For this review, use the dimensioned drawing (mm, ordinates from the lowest corner) and the shaded views. Coordinates: 2 decimals unless noted, no trailing zeros. Write each loop counter-clockwise with the first axis right and the second up, starting at its lowest first coordinate (ties: lowest second). Pieces come first, ordered by that corner, then holes. Notation, with made-up numbers: (2, 80.5) - (33, 80.5) arc R22 ccw to (33, 87.5) - close; hole circle Ø5 at (29.25, 29). An arc over 180 degrees is marked (long way). One line per item, written item: value.
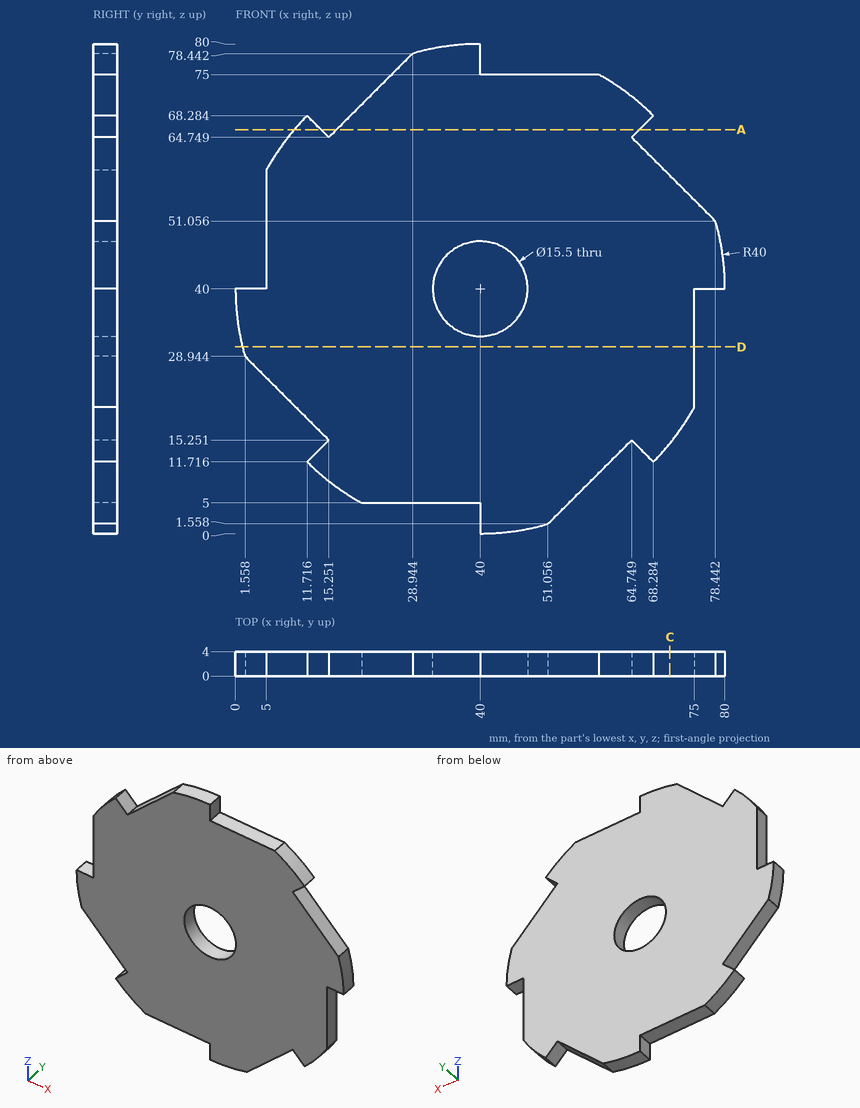
1. Consider section D-D, the plane z = 30.5. Write out the cut boundary in (x, y) (1 decimal).
Answer block:
outline: (1.1, 0) - (75, 0) - (75, 4) - (1.1, 4) - close
2. Insertion check: pin 1 Ø2 at (y, z) = (1.5, 52) entering from -X; pin 2 Ø1 at (x, y) = (36.5, 2.5) entering from -Z; pin 3 Ø1.2 at (y, z) = (1.5, 3.5) entering from -X. Each pin has a flat end and moves straight along its axis. Give the tip position at first contact, or say it passes through.
Answer block:
pin 1: stops at x = 5
pin 2: stops at z = 5
pin 3: stops at x = 40
3. Consider section C-C, the plane x = 71. Write out the cut boundary in (y, z).
Answer block:
outline: (0, 14.72) - (4, 14.72) - (4, 58.5) - (0, 58.5) - close
4. Consider section A-A, the plane z = 66. Write out the cut boundary in (x, y).
Answer block:
outline: (9.6, 0) - (14, 0) - (14, 4) - (9.6, 4) - close; (16.5, 0) - (66, 0) - (66, 4) - (16.5, 4) - close
5. Wall thickness on line 1 along Z through (x, y) = (39.5, 1.7); line 2 along X through (y, z) = (1.4, 36.5) (1 decimal): over which ranges is each line inside the solid? List them lowest first.
Answer block:
line 1: z = 5 to 32.27, 47.73 to 80
line 2: x = 0.2 to 33.1, 46.9 to 75
